Input: part model. Units: mm. Frame: model coordinates. Face numbers are marked on the shaded views. A direction names the side the tool comes from. Give positions to 0.01 mm unless a question says otherwise; leave off trailing zeros. Loops run counter-clockwise (first coordinate to the right, second up) from the corner with the lowest first, then second, coordinate; pieces in that order, holes last. Notation, with made-up numbers: M 55.25,13.5 L 77.25,13.5 A25 ccw 77.25,49.5 Z; hole C -16,-26 d9. An arc over 180 degrees is marked long. One line per item, written item: value. Start each with the question number.
(1) Pin query (flat end, axial travel): P1, Ø0.8, axis at y = 1.5, z = 17.5, coming from the -X side; P2, Ø0.5, axis at y = 1.5, z = 17.5, coming from the +X side; P3, Ø1, axis at y = 0, z = 11, coming from the -X side; P4, Ø4, axis at x = 0, y = -1, coming from the +Z side. Return the tip coordinate at first contact, or that it passes through.
(2) Section C-C on z = 6.5. Output: boundary loops of the cut face in (x, y), plus the area to 3 significant figures.
(3) Ray query, line 1 along Z through (x, y) = (-1.25, 0.25); line 2 along Y through (x, z) = (1.5, 10.5); line 3 along X through (y, z) = (0.5, 10.5). Return the intervals inside material, ascending. Write a range as from..to.
(4) Section A-A on y = 0. Output: boundary loops of the cut face in (x, z), plus the area to 3 significant figures.
(5) Access query for the marked faces 1 and 2. Directions: +Z, -Z, +X, -X, +Y, -Y. A direction counts if a zero-diameter tool reaches every point of the face in a straight line with its end or side. Return the directions, or none.
Solid Edge part; units mm, degrees
sketch "Sketch1" plane through (0, 0, 0) normal (0, -1, 0) x (1, 0, 0)
  line L0 (0, 0) -> (0, 18)
  line L1 (0, 18) -> (4, 18)
  line L2 (4, 18) -> (4, 14.5)
  line L3 (4, 14.5) -> (2.5, 14.5)
  line L4 (2.5, 0) -> (2.5, 14.5)
  line L5 (0, 0) -> (2.5, 0)
revolve "RevolvedProtrusion1" add sketch "Sketch1" angle 360 about axis through (0, 0, 0) along (0, 0, 1)
chamfer "Chamfer1" distance 0.5 angle 45 1 edges at (-2.5, 0, 0)
cosmetic_thread "Thread1"
fillet "Lekerekítés_1" radius 1.8 1 edges at (-4, 0, 18)
fillet "Lekerekítés_3" radius 0.2 1 edges at (-4, 0, 14.5)
sketch "Sketch2" plane through (0, 0, 18) normal (0, 0, 1) x (0, -1, 0)
  line L0 (0, -2.5) -> (0.5, -2.5)
  line L1 (0.5, -2.5) -> (0.5, -0.7199)
  arc A0 (0.7199, -0.5) -> (0.5, -0.7199) centre (0.7199, -0.7199) ccw
  line L2 (0.7199, -0.5) -> (2.5, -0.5)
  line L3 (2.5, 0) -> (2.5, -0.5)
  line L4 (2.5, 0) -> (2.5, 0.5)
  line L5 (0.7371, 0.5) -> (2.5, 0.5)
  arc A1 (0.7371, 0.5) -> (0.5, 0.7371) centre (0.7371, 0.7371) cw
  line L6 (0.5, 0.7371) -> (0.5, 2.5)
  line L7 (0, 2.5) -> (0.5, 2.5)
  line L8 (0, 2.5) -> (-0.5, 2.5)
  line L9 (-0.5, 0.7495) -> (-0.5, 2.5)
  arc A2 (-0.5, 0.7495) -> (-0.7495, 0.5) centre (-0.7495, 0.7495) cw
  line L10 (-2.5, 0.5) -> (-0.7495, 0.5)
  line L11 (-2.5, 0) -> (-2.5, 0.5)
  line L12 (-2.5, 0) -> (-2.5, -0.5)
  line L13 (-2.5, -0.5) -> (-0.7175, -0.5)
  arc A3 (-0.5, -0.7175) -> (-0.7175, -0.5) centre (-0.7175, -0.7175) ccw
  line L14 (-0.5, -2.5) -> (-0.5, -0.7175)
  line L15 (0, -2.5) -> (-0.5, -2.5)
extrude "Kivágás_1" cut sketch "Sketch2" against normal blind 1.5
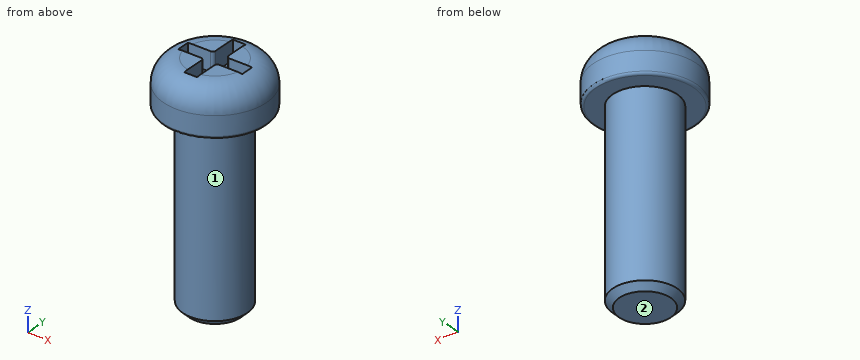
Output values:
1. P1: stops at x = -3.49
1. P2: stops at x = 3.37
1. P3: stops at x = -2.5
1. P4: stops at z = 18
2. outline: C 0,0 d5
2. area: 19.6 mm²
3. line 1: z = 0..16.5
3. line 2: y = -2..2
3. line 3: x = -2.45..2.45
4. outline: M -4,14.7 A0.2 ccw -3.8,14.5 L -2.5,14.5 L -2.5,0.5 L -2,0 L 2,0 L 2.5,0.5 L 2.5,14.5 L 3.8,14.5 A0.2 ccw 4,14.7 L 4,16.2 A1.8 ccw 2.5,17.97 L 2.5,16.5 L -2.5,16.5 L -2.5,17.97 A1.8 ccw -4,16.2 Z
4. area: 91.3 mm²
5. face 1: -Z
5. face 2: -Z, +X, -X, +Y, -Y
